from build123d import *


with BuildPart() as part:
    # Sketch1 → Revolve1 (revolve)
    with BuildSketch(Plane.XY, mode=Mode.PRIVATE) as revolve1_sk:
        Polygon((1.7145, 0), (5, 0), (4.3235, 0.5), (5, 1), (4.3235, 1.5), (5, 2), (4.3235, 2.5), (5, 3), (4.3235, 3.5), (5, 4), (4.3235, 4.5), (5, 5), (4.3235, 5.5), (5, 6), (4.3235, 6.5), (5, 7), (4.3235, 7.5), (5, 8), (4.3235, 8.5), (5, 9), (4.3235, 9.5), (5, 10), (4.3235, 10.5), (5, 11), (4.3235, 11.5), (5, 12), (4.3235, 12.5), (5, 13), (4.3235, 13.5), (5, 14), (4.3235, 14.5), (5, 15), (4.3235, 15.5), (5, 16), (4.3235, 16.5), (5, 17), (4.3235, 17.5), (5, 18), (4.3235, 18.5), (5, 19), (4.3235, 19.5), (5, 20), (4.3235, 20.5), (5, 21), (4.3235, 21.5), (5, 22), (4.3235, 22.5), (5, 23), (4.3235, 23.5), (5, 24), (4.3235, 24.5), (5, 25), (4.3235, 25.5), (5, 26), (4.3235, 26.5), (5, 27), (4.3235, 27.5), (5, 28), (1.7145, 28), (1.5875, 27.873), (1.5875, 0.127), align=None)
    revolve(revolve1_sk.sketch.rotate(Axis((0, 0, 0), (0, 1, 0)), 90), axis=Axis((0, 0, 0), (0, 1, 0)))  # turned: the seam where the file's is


solid = part.part
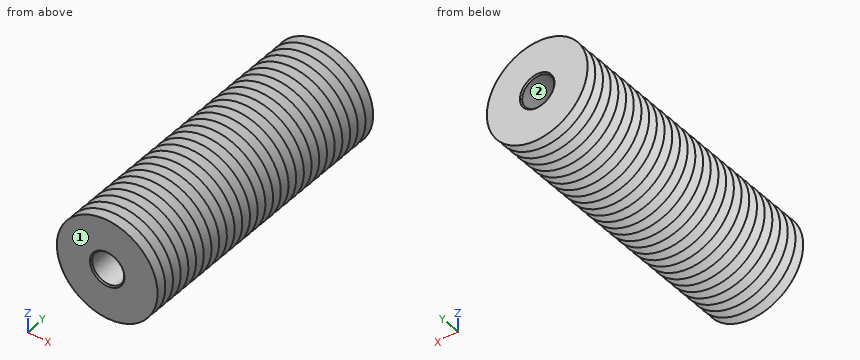
Can you work these out from the model? Positions are in its coordinate system, mm. Face numbers are marked on the shaded views. Coordinates: 2 decimals unless noted, no trailing zeros. Answer as a JSON object with one key per item and string values. Group by question number.
Q1. I need wall thicknesses on line 1 (Z direction, x = 1, y = 19.25); line 2 (X direction, y = 11.25, z = -0.5); line 3 (Z direction, x = 3.75, y = 4.75). Which ranges of each line are inside material? Lowest first, please. Write a range as from..to.
Q2. Will these pins go through, and if not, where does the flat tip stop? P1, Ø1.9, axis at x = 0, z = 0, coming from the -Y side; P2, Ø2, axis at y = 21, z = 1.5, coming from the -X side; P3, Ø1, axis at y = 9.5, z = 2.5, coming from the -X side; P4, Ø1.5, axis at x = 3, y = 5.5, coming from the -Z side.
Q3. We'd pull the mould along X, two halves only. Please class the marked faces 1 and 2: +X half, -X half, draft (parallel to the pull), parting line (faces both ways), or undercut.
Determined:
{
 "1": {"line 1": "z = -4.55..-1.23, 1.23..4.55", "line 2": "x = -4.63..-1.51, 1.51..4.63", "line 3": "z = -2.77..2.77"},
 "2": {"P1": "passes through", "P2": "stops at x = -4.97", "P3": "stops at x = -4.38", "P4": "stops at z = -4.36"},
 "3": {"face 1": "draft", "face 2": "undercut"}
}
